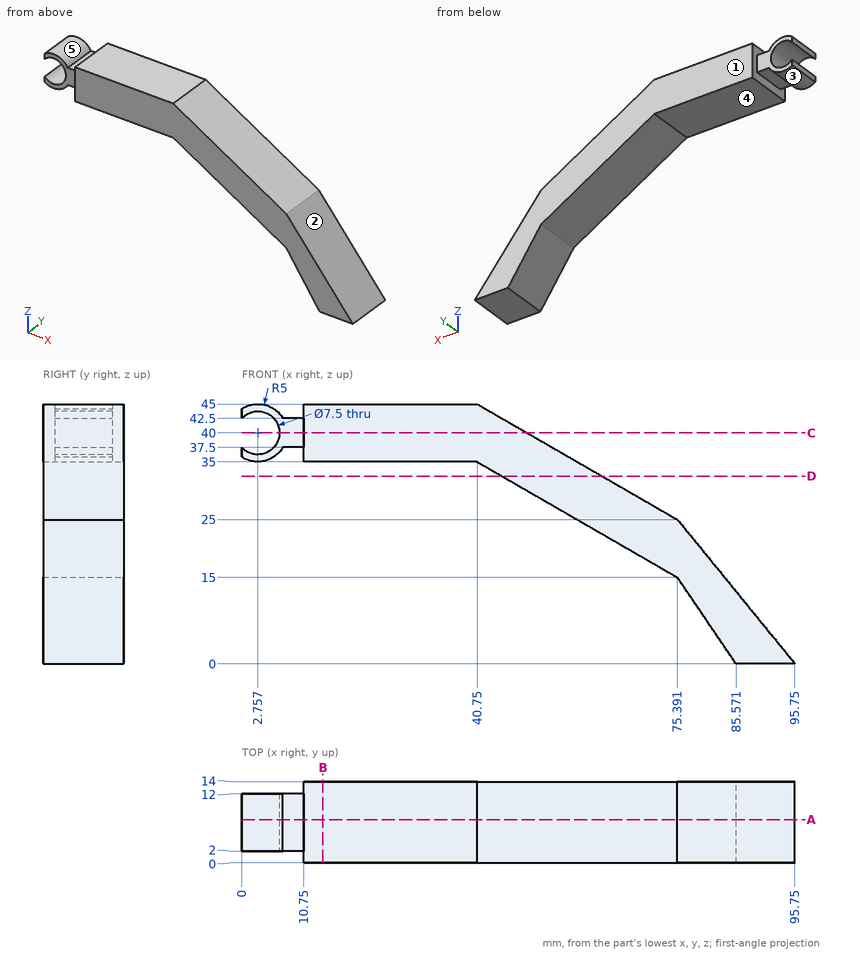
Check sheet for the drawn part. Datum: minimum x, y, z corner. Units: mm. A direction names the side the tool comes from. Give positions to 0.01 mm unless a question says otherwise; leave off trailing zeros. Write each loop counter-clockwise with the first axis right and the second up, starting at its lowest first coordinate (ties: lowest second). Pieces come first, ordered by that corner, then holes.
(1) Cross-section at C-C (z = 40). Enter the section's corners in (x, y).
(2) Mould release check, pull along X, two halves, no side actions. Record for the marked faces 1, 2 and 3: +X half, -X half, draft (parallel to the pull), parting line (faces both ways), or undercut.
(3) Cross-section at A-A (y = 7.5). Enter the section's corners in (x, z).
(4) Gauge pin test, flat ends, axial feed: pin 1 (2 mm diameter, centred on x = 85, y = 6, fed in from +Z); pin 2 (12 mm diameter, centred on x = 2.76, z = 40, fed in from +Y); pin 3 (10 mm diameter, centred on x = 68.5, z = 37.5, fed in from -Y); pin 4 (8 mm diameter, centred on x = 3.5, z = 41, fed in from -Y). Record the tip position at first contact, or that the pin passes through.
(5) Material ranges on line 1 (Z direction, x = 32, y = 1.5); line 2 (Z direction, x = 82, y = 3.75) (1 decimal); line 3 (X direction, y = 4, z = 16.5) (1 decimal), recorded low to high.
(6) Access from +Z, -Z, +X, -X, +Y, -Y to the whole of each face (thin tool, end or side, straight path). Record for the marked faces 4 and 5.
(7) Cross-section at D-D (z = 32.5). Enter the section's corners in (x, y).
(8) Cross-section at B-B (x = 14). Enter the section's corners in (y, z), plus the area to 3 significant figures.
Worked out:
1. outline: (6.51, 2) - (10.75, 2) - (10.75, 0) - (49.41, 0) - (49.41, 14) - (10.75, 14) - (10.75, 12) - (6.51, 12) - close
2. face 1: draft
2. face 2: +X half
2. face 3: undercut
3. outline: (0, 35.83) arc R5 ccw to (7.09, 37.5) - (10.75, 37.5) - (10.75, 35) - (40.75, 35) - (75.39, 15) - (85.57, 0) - (95.75, 0) - (75.39, 25) - (40.75, 45) - (10.75, 45) - (10.75, 42.5) - (7.09, 42.5) arc R5 ccw to (0, 44.17) - (0, 42.54) arc R3.75 cw (long way) to (0, 37.46) - close
4. pin 1: stops at z = 14.43
4. pin 2: stops at y = 12
4. pin 3: passes through
4. pin 4: stops at y = 2
5. line 1: z = 35 to 45
5. line 2: z = 5.3 to 16.9
5. line 3: x = 72.8 to 82.3
6. face 4: -Z, -X, +Y, -Y
6. face 5: +Z, +Y, -Y
7. outline: (45.08, 0) - (62.4, 0) - (62.4, 14) - (45.08, 14) - close
8. outline: (0, 35) - (14, 35) - (14, 45) - (0, 45) - close
8. area: 140 mm2
